Here's how the part is built. I have some questions about the finished solid (model axes, mm). A direction names the side the tool comes from. Give positions to 0.01 mm unless a question says otherwise; leave off trailing zeros. Loops run counter-clockwise (first coordinate to the right, second up) from the corner with the lowest first, then second, coordinate; pieces in that order, holes last. Notation, with made-up numbers: (-1.5, 0.5) -> (31.5, 0.5) arc R11 cw to (31.5, 12.5) -> close; hole circle Ø10 at (17.25, -33.75). An arc over 180 degrees is marked (long way). Answer in a Markdown table with one row per item. Add a question column.
Item 1: If we section it at B-B (x = 0): Write out the boundary of the cut face in (y, z) (3 decimals).
Item 2: If I drill on line 1 (Z direction, x = 0, y = -2.1) (3 decimals); line 2 (X direction, y = -0.7, z = 1.7); line 3 (X direction, y = -2.9, z = 0.15), over which ranges is the centre line in solid material (lowest first)?
Item 3: Which directions (+Z, -Z, +X, -X, +Y, -Y) give clear straight access to the entire face, cutting with the end or side of a thin tool? Please do faces 1 (the face through (0, -2, -1.905)), 2 (the face through (-4.318, -1, 0)).
Item 4: If we section it at A-A (z = 0): Write out the boundary of the cut face in (x, y), then the cut area to 3 significant figures.
Item 5: If we section it at D-D (y = -2.55): Write out the boundary of the cut face in (x, z) (3 decimals).
Item 6: If we section it at C-C (y = -0.7): Write out the boundary of the cut face in (x, z) (1 decimal).
```python
from build123d import *

# Parameters (mm, degrees)
F1_DEPTH = 3.81
F2_R     = 0.5
F3_DEPTH = 25.4
F5_DEPTH = 1.27


# Not quite as in the source:
# - ends of sketch curves that miss each other by under 0.0002 mm in the source are joined


with BuildPart() as f1:
    # F0 (on Front) → F1 (new body)
    with BuildSketch(Plane.XZ):
        with BuildLine():
            Line((9.9798112172, 1.905), (-9.9798084652, 1.905))
            ThreePointArc((-9.9798084652, 1.905), (-10.16, 0), (-9.9798084652, -1.9049994747))
            Line((-9.9798084652, -1.9049994747), (9.9798084652, -1.905))
            ThreePointArc((9.9798084652, -1.905), (10.16, 0), (9.9798112172, 1.905))
        make_face()
    extrude(amount=F1_DEPTH)

    # F2 (on face) → F3 (cut)
    with BuildSketch(Plane.XZ.offset(3.81)):
        Circle(F2_R)
    extrude(amount=-F3_DEPTH, mode=Mode.SUBTRACT)

    # F4 (on face) → F5 (cut)
    with BuildSketch(Plane.XZ):
        Polygon((7.1755, 1.905), (4.318, 1.905), (4.318, -0.0512809254), (4.318, -1.905), (7.1755, -1.905), align=None)
        Polygon((-4.318, 0), (-4.318, 1.905), (-7.1755, 1.905), (-7.1755, -1.905), (-4.318, -1.905), align=None)
    extrude(amount=F5_DEPTH, mode=Mode.SUBTRACT)


solid = f1.part
```
Recorded:
| question | item | result |
|---|---|---|
| 1 | outline | (-3.81, -1.905) -> (0, -1.905) -> (0, -0.5) -> (-3.81, -0.5) -> close; (-3.81, 0.5) -> (0, 0.5) -> (0, 1.905) -> (-3.81, 1.905) -> close |
| 2 | line 1 | z = -1.905 to -0.5, 0.5 to 1.905 |
| 2 | line 2 | x = -10.02 to -7.18, -4.32 to 4.32, 7.18 to 10.02 |
| 2 | line 3 | x = -10.16 to -0.48, 0.48 to 10.16 |
| 3 | face 1 | -Z, +X, -X, +Y, -Y |
| 3 | face 2 | +Z, -Z, +Y |
| 4 | outline | (-10.16, -3.81) -> (-0.5, -3.81) -> (-0.5, 0) -> (-4.32, 0) -> (-4.32, -1.27) -> (-7.18, -1.27) -> (-7.18, 0) -> (-10.16, 0) -> close; (0.5, -3.81) -> (10.16, -3.81) -> (10.16, 0) -> (7.18, 0) -> (7.18, -1.27) -> (4.32, -1.27) -> (4.32, 0) -> (0.5, 0) -> close |
| 4 | area | 66.4 mm^2 |
| 5 | outline | (-9.98, -1.905) -> (9.98, -1.905) arc R10.16 ccw to (9.98, 1.905) -> (-9.98, 1.905) arc R10.16 ccw to start; hole circle Ø1 at (0, 0) |
| 6 | outline | (-10, -1.9) -> (-7.2, -1.9) -> (-7.2, 1.9) -> (-10, 1.9) arc R10.2 ccw to start; (-4.3, -1.9) -> (4.3, -1.9) -> (4.3, 1.9) -> (-4.3, 1.9) -> close; (7.2, -1.9) -> (10, -1.9) arc R10.2 ccw to (10, 1.9) -> (7.2, 1.9) -> close; hole circle Ø1 at (0, 0) |
